Build history of the part. All positions in model axes, mm. A direction names the side the tool comes from. Round coordinates to 2 decimals unless told otherwise and drop trailing zeros. Loops run counter-clockwise (first coordinate to the right, second up) from the corner with the lowest first, then second, coordinate; pieces in that order, holes last. Notation, with made-up numbers: (25, 86.25) -> (41, 86.25) arc R15 ccw to (41, 99.25) -> close; hole circle Ø1 at (55.5, -9.5). An arc over 180 degrees is marked (long way). Put each result on its own line as item: value. Start each with the question number.
Item 1: Cut at C-C, the plane x = 1. List the corners of the cut face in (y, z).
Item 2: Cut at A-A, the plane z = 0. List the corners of the cut face in (x, y), plus the area to 3 significant figures.
Item 3: Drill centre lines: probe 1 along X at (y, z) = (2.75, 5); probe 2 along Y at (x, z) = (12, -1.25); probe 3 along Z at (x, y) = (15.5, -9.25). Where is each one in solid material? Low to high. Write a range as [from, to].
Item 4: Cut at D-D, the plane z = -3.25. List the corners of the cut face in (x, y).
Item 5: Pull direction X, two halves, no side cores. Call faces 3 (the flat face through (6.4, -3.8, -6.35)), 4 (the cylindrical face through (15.13, -8.71, -0.56)), 5 (the flat face through (10.319, -4, 0)): +X half, -X half, draft (parallel to the pull), parting line (faces both ways), or undercut.
Item 6: Tool access for faces 1 (the flat face through (15, -7.144, 2)), 2 (the flat face through (23.195, -9, 0)): list every direction of +Z, -Z, +X, -X, +Y, -Y with a clear straight run to the whole face (end or side of a thin tool).
Item 7: Cut at B-B, the plane y = 4.5. List the corners of the cut face in (x, z), plus the area to 3 significant figures.
Item 8: Flat gauge pins, fed straight in: pin 1 Ø3 at (x, y) = (3, -5.5) entering from +Z; pin 2 Ø4 at (x, z) = (17.66, 0) entering from +Y; pin 3 Ø2 at (y, z) = (-5, -1.5) entering from +X; pin 4 Ø3 at (y, z) = (4, -3.5) entering from +X. Where does each tip first touch, or does it go through?
```python
from build123d import *

# Parameters (mm, degrees)
SKETCH1_R           = 7.14375
BOSS_EXTRUDE1_DEPTH = 6.35
SKETCH2_R           = 2.5908
CUT_EXTRUDE1_DEPTH  = 11.31875


with BuildPart() as part:
    # Sketch1 → Boss-Extrude1 (new body, symmetric)
    with BuildSketch(Plane.XY):
        with BuildLine():
            Line((0, -10.31875), (23.19528, -10.31875))
            Line((23.19528, -10.31875), (23.19528, -7.14375))
            Line((23.19528, -7.14375), (10.31875, -7.14375))
            Line((10.31875, -7.14375), (10.31875, 0))
            ThreePointArc((10.31875, 0), (-7.296458098, 7.296458098), (0, -10.31875))
        make_face()
        Circle(SKETCH1_R, mode=Mode.SUBTRACT)
    extrude(amount=BOSS_EXTRUDE1_DEPTH, both=True)

    # Sketch2 → Cut-Extrude1 (cut, through all)
    with BuildSketch(Plane(origin=(0, 0, 0), x_dir=(1, 0, 0), z_dir=(0, 1, 0))):
        with Locations(Location((17.65808, 0, 0), (0, 0, 270))):  # turned: the seam where the file's is
            Circle(SKETCH2_R)
    extrude(amount=-CUT_EXTRUDE1_DEPTH, mode=Mode.SUBTRACT)


solid = part.part
```
Reply:
1. outline: (-10.32, -6.35) -> (-7.07, -6.35) -> (-7.07, 6.35) -> (-10.32, 6.35) -> close; (7.07, -6.35) -> (10.27, -6.35) -> (10.27, 6.35) -> (7.07, 6.35) -> close
2. outline: (0, -10.32) -> (15.07, -10.32) -> (15.07, -7.14) -> (10.32, -7.14) -> (10.32, 0) arc R10.32 ccw (long way) to start; (20.25, -10.32) -> (23.2, -10.32) -> (23.2, -7.14) -> (20.25, -7.14) -> close; hole circle Ø14.29 at (0, 0)
2. area: 221 mm^2
3. probe 1: x = [-9.95, -6.59], [6.59, 9.95]
3. probe 2: y = [-10.32, -7.14]
3. probe 3: z = [-6.35, -1.43], [1.43, 6.35]
4. outline: (0, -10.32) -> (23.2, -10.32) -> (23.2, -7.14) -> (10.32, -7.14) -> (10.32, 0) arc R10.32 ccw (long way) to start; hole circle Ø14.29 at (0, 0)
5. face 3: draft
5. face 4: undercut
5. face 5: +X half
6. face 1: +Z, -Z, +X, +Y
6. face 2: +Z, -Z, +X, +Y, -Y
7. outline: (-9.29, -6.35) -> (-5.55, -6.35) -> (-5.55, 6.35) -> (-9.29, 6.35) -> close; (5.55, -6.35) -> (9.29, -6.35) -> (9.29, 6.35) -> (5.55, 6.35) -> close
7. area: 94.9 mm^2
8. pin 1: stops at z = 6.35
8. pin 2: passes through
8. pin 3: stops at x = 10.32
8. pin 4: stops at x = 10.01
